from build123d import *

# Parameters (mm, degrees)
IZIM2_R                           = 5
KES_EKSTR_ZYON3_DEPTH             = 12
KES_EKSTR_ZYON3_TAPER             = -20
KES_EKSTR_ZYON3_OTHER_WAY_DEPTH   = 12
KES_EKSTR_ZYON3_OTHER_WAY_DRAFT   = -20
DAIRESEL_KAPLAMA1_COUNT           = 5
DAIRESEL_KAPLAMA1_COPY_1_SKETCH_R = 5
DAIRESEL_KAPLAMA1_COPY_1_DEPTH    = 12
DAIRESEL_KAPLAMA1_COPY_1_DRAFT    = -20
DAIRESEL_KAPLAMA1_COPY_2_SKETCH_R = 5
DAIRESEL_KAPLAMA1_COPY_2_DEPTH    = 12
DAIRESEL_KAPLAMA1_COPY_2_DRAFT    = -20
DAIRESEL_KAPLAMA1_COPY_3_SKETCH_R = 5
DAIRESEL_KAPLAMA1_COPY_3_DEPTH    = 12
DAIRESEL_KAPLAMA1_COPY_3_DRAFT    = -20
DAIRESEL_KAPLAMA1_COPY_4_SKETCH_R = 5
DAIRESEL_KAPLAMA1_COPY_4_DEPTH    = 12
DAIRESEL_KAPLAMA1_COPY_4_DRAFT    = -20
DAIRESEL_KAPLAMA1_COPY_5_SKETCH_R = 5
DAIRESEL_KAPLAMA1_COPY_5_DEPTH    = 12
DAIRESEL_KAPLAMA1_COPY_5_DRAFT    = -20
DAIRESEL_KAPLAMA1_COPY_6_SKETCH_R = 5
DAIRESEL_KAPLAMA1_COPY_6_DEPTH    = 12
DAIRESEL_KAPLAMA1_COPY_6_DRAFT    = -20
DAIRESEL_KAPLAMA1_COPY_7_SKETCH_R = 5
DAIRESEL_KAPLAMA1_COPY_7_DEPTH    = 12
DAIRESEL_KAPLAMA1_COPY_7_DRAFT    = -20
DAIRESEL_KAPLAMA1_COPY_8_SKETCH_R = 5
DAIRESEL_KAPLAMA1_COPY_8_DEPTH    = 12
DAIRESEL_KAPLAMA1_COPY_8_DRAFT    = -20


with BuildPart() as part:
    # Çizim1 → Döndür1 (revolve)
    with BuildSketch(Plane.XY, mode=Mode.PRIVATE) as d_nd_r1_sk:
        Polygon((-10.136635142, 50), (-0.136635142, 40), (9.863364858, 50), (11.863364858, 50), (11.863364858, 20), (14.863364858, 20), (14.863364858, 15), (11.863364858, 15), (-12.136635142, 15), (-15.136635142, 15), (-15.136635142, 20), (-12.136635142, 20), (-12.136635142, 50), align=None)
    revolve(d_nd_r1_sk.sketch.rotate(Axis((-17.676704828, 0, 0), (1, 0, 0)), 90), axis=Axis((-17.676704828, 0, 0), (1, 0, 0)))

    # Çizim2 → Kes-Ekstrüzyon3 (cut)
    with BuildSketch(Plane(origin=(-0.136635142, 0, 0), x_dir=(0, 0, -1), z_dir=(1, 0, 0))):
        with Locations((0, 30)):
            Circle(IZIM2_R)
    kes_ekstr_zyon3 = extrude(amount=-KES_EKSTR_ZYON3_DEPTH, taper=KES_EKSTR_ZYON3_TAPER, mode=Mode.SUBTRACT)


with BuildPart() as kes_ekstr_zyon3_other_way_tool:
    # Çizim2 → Kes-Ekstrüzyon3 other way (with draft: the straight prism first)
    with BuildSketch(Plane(origin=(-0.136635142, 0, 0), x_dir=(0, 0, -1), z_dir=(1, 0, 0))):
        with Locations((0, 30)):
            Circle(IZIM2_R)
    extrude(amount=KES_EKSTR_ZYON3_OTHER_WAY_DEPTH)
    # Kes-Ekstrüzyon3 other way: the draft: its side faces are tilted about the plane it starts from
    kes_ekstr_zyon3_other_way_sides = [kes_ekstr_zyon3_other_way_tool.faces().sort_by_distance(p)[0] for p in [
        (5.863364858, 30, 5),
    ]]
    draft(kes_ekstr_zyon3_other_way_sides, Plane(origin=(-0.136635142, 0, 0), x_dir=(0, 0, -1), z_dir=(1, 0, 0)), KES_EKSTR_ZYON3_OTHER_WAY_DRAFT)


with BuildPart() as part_1:
    add(part.part)

    # Kes-Ekstrüzyon3 other way: cut by kes_ekstr_zyon3_other_way_tool
    add(kes_ekstr_zyon3_other_way_tool.part, mode=Mode.SUBTRACT)

    # Dairesel Kaplama1: Kes-Ekstrüzyon3 ×5 about axis
    dairesel_kaplama1_axis = Axis((0, 0, 0), (1, 0, 0))
    for i in range(1, DAIRESEL_KAPLAMA1_COUNT):
        add(kes_ekstr_zyon3.rotate(dairesel_kaplama1_axis, i * 360 / DAIRESEL_KAPLAMA1_COUNT), mode=Mode.SUBTRACT)


with BuildPart() as dairesel_kaplama1_copy_1_tool:
    # Dairesel Kaplama1 copy 1 sketch → Dairesel Kaplama1 copy 1 (with draft: the straight prism first)
    with BuildSketch(Plane(origin=(-0.136635142, 0, 0), x_dir=(0, 0.9510565162951535, -0.30901699437494745), z_dir=(1, 0, 0))):
        with Locations((0, 30)):
            Circle(DAIRESEL_KAPLAMA1_COPY_1_SKETCH_R)
    extrude(amount=DAIRESEL_KAPLAMA1_COPY_1_DEPTH)
    # Dairesel Kaplama1 copy 1: the draft: its side faces are tilted about the plane it starts from
    dairesel_kaplama1_copy_1_sides = [dairesel_kaplama1_copy_1_tool.faces().sort_by_distance(p)[0] for p in [
        (5.863364858, 4.51522725, 30.076780461),
    ]]
    draft(dairesel_kaplama1_copy_1_sides, Plane(origin=(-0.136635142, 0, 0), x_dir=(0, 0.9510565162951535, -0.30901699437494745), z_dir=(1, 0, 0)), DAIRESEL_KAPLAMA1_COPY_1_DRAFT)


with BuildPart() as part_2:
    add(part_1.part)

    # Dairesel Kaplama1 copy 1: cut by dairesel_kaplama1_copy_1_tool
    add(dairesel_kaplama1_copy_1_tool.part, mode=Mode.SUBTRACT)


with BuildPart() as dairesel_kaplama1_copy_2_tool:
    # Dairesel Kaplama1 copy 2 sketch → Dairesel Kaplama1 copy 2 (with draft: the straight prism first)
    with BuildSketch(Plane(origin=(-0.136635142, 0, 0), x_dir=(0, 0.5877852522924732, 0.8090169943749473), z_dir=(1, 0, 0))):
        with Locations((0, 30)):
            Circle(DAIRESEL_KAPLAMA1_COPY_2_SKETCH_R)
    extrude(amount=DAIRESEL_KAPLAMA1_COPY_2_DEPTH)
    # Dairesel Kaplama1 copy 2: the draft: its side faces are tilted about the plane it starts from
    dairesel_kaplama1_copy_2_sides = [dairesel_kaplama1_copy_2_tool.faces().sort_by_distance(p)[0] for p in [
        (5.863364858, -27.209436093, 13.588472597),
    ]]
    draft(dairesel_kaplama1_copy_2_sides, Plane(origin=(-0.136635142, 0, 0), x_dir=(0, 0.5877852522924732, 0.8090169943749473), z_dir=(1, 0, 0)), DAIRESEL_KAPLAMA1_COPY_2_DRAFT)


with BuildPart() as part_3:
    add(part_2.part)

    # Dairesel Kaplama1 copy 2: cut by dairesel_kaplama1_copy_2_tool
    add(dairesel_kaplama1_copy_2_tool.part, mode=Mode.SUBTRACT)


with BuildPart() as dairesel_kaplama1_copy_3_tool:
    # Dairesel Kaplama1 copy 3 sketch → Dairesel Kaplama1 copy 3 (with draft: the straight prism first)
    with BuildSketch(Plane(origin=(-0.136635142, 0, 0), x_dir=(0, -0.587785252292473, 0.8090169943749476), z_dir=(1, 0, 0))):
        with Locations((0, 30)):
            Circle(DAIRESEL_KAPLAMA1_COPY_3_SKETCH_R)
    extrude(amount=DAIRESEL_KAPLAMA1_COPY_3_DEPTH)
    # Dairesel Kaplama1 copy 3: the draft: its side faces are tilted about the plane it starts from
    dairesel_kaplama1_copy_3_sides = [dairesel_kaplama1_copy_3_tool.faces().sort_by_distance(p)[0] for p in [
        (5.863364858, -21.33158357, -21.678642541),
    ]]
    draft(dairesel_kaplama1_copy_3_sides, Plane(origin=(-0.136635142, 0, 0), x_dir=(0, -0.587785252292473, 0.8090169943749476), z_dir=(1, 0, 0)), DAIRESEL_KAPLAMA1_COPY_3_DRAFT)


with BuildPart() as part_4:
    add(part_3.part)

    # Dairesel Kaplama1 copy 3: cut by dairesel_kaplama1_copy_3_tool
    add(dairesel_kaplama1_copy_3_tool.part, mode=Mode.SUBTRACT)


with BuildPart() as dairesel_kaplama1_copy_4_tool:
    # Dairesel Kaplama1 copy 4 sketch → Dairesel Kaplama1 copy 4 (with draft: the straight prism first)
    with BuildSketch(Plane(origin=(-0.136635142, 0, 0), x_dir=(0, -0.9510565162951536, -0.30901699437494723), z_dir=(1, 0, 0))):
        with Locations((0, 30)):
            Circle(DAIRESEL_KAPLAMA1_COPY_4_SKETCH_R)
    extrude(amount=DAIRESEL_KAPLAMA1_COPY_4_DEPTH)
    # Dairesel Kaplama1 copy 4: the draft: its side faces are tilted about the plane it starts from
    dairesel_kaplama1_copy_4_sides = [dairesel_kaplama1_copy_4_tool.faces().sort_by_distance(p)[0] for p in [
        (5.863364858, 14.025792413, -26.986610517),
    ]]
    draft(dairesel_kaplama1_copy_4_sides, Plane(origin=(-0.136635142, 0, 0), x_dir=(0, -0.9510565162951536, -0.30901699437494723), z_dir=(1, 0, 0)), DAIRESEL_KAPLAMA1_COPY_4_DRAFT)


with BuildPart() as part_5:
    add(part_4.part)

    # Dairesel Kaplama1 copy 4: cut by dairesel_kaplama1_copy_4_tool
    add(dairesel_kaplama1_copy_4_tool.part, mode=Mode.SUBTRACT)


with BuildPart() as dairesel_kaplama1_copy_5_tool:
    # Dairesel Kaplama1 copy 5 sketch → Dairesel Kaplama1 copy 5 (with draft: the straight prism first)
    with BuildSketch(Plane(origin=(-0.136635142, 0, 0), x_dir=(0, 0.9510565162951535, -0.30901699437494745), z_dir=(1, 0, 0))):
        with Locations((0, 30)):
            Circle(DAIRESEL_KAPLAMA1_COPY_5_SKETCH_R)
    extrude(amount=DAIRESEL_KAPLAMA1_COPY_5_DEPTH)
    # Dairesel Kaplama1 copy 5: the draft: its side faces are tilted about the plane it starts from
    dairesel_kaplama1_copy_5_sides = [dairesel_kaplama1_copy_5_tool.faces().sort_by_distance(p)[0] for p in [
        (5.863364858, 4.51522725, 30.076780461),
    ]]
    draft(dairesel_kaplama1_copy_5_sides, Plane(origin=(-0.136635142, 0, 0), x_dir=(0, 0.9510565162951535, -0.30901699437494745), z_dir=(1, 0, 0)), DAIRESEL_KAPLAMA1_COPY_5_DRAFT)


with BuildPart() as part_6:
    add(part_5.part)

    # Dairesel Kaplama1 copy 5: cut by dairesel_kaplama1_copy_5_tool
    add(dairesel_kaplama1_copy_5_tool.part, mode=Mode.SUBTRACT)


with BuildPart() as dairesel_kaplama1_copy_6_tool:
    # Dairesel Kaplama1 copy 6 sketch → Dairesel Kaplama1 copy 6 (with draft: the straight prism first)
    with BuildSketch(Plane(origin=(-0.136635142, 0, 0), x_dir=(0, 0.5877852522924732, 0.8090169943749473), z_dir=(1, 0, 0))):
        with Locations((0, 30)):
            Circle(DAIRESEL_KAPLAMA1_COPY_6_SKETCH_R)
    extrude(amount=DAIRESEL_KAPLAMA1_COPY_6_DEPTH)
    # Dairesel Kaplama1 copy 6: the draft: its side faces are tilted about the plane it starts from
    dairesel_kaplama1_copy_6_sides = [dairesel_kaplama1_copy_6_tool.faces().sort_by_distance(p)[0] for p in [
        (5.863364858, -27.209436093, 13.588472597),
    ]]
    draft(dairesel_kaplama1_copy_6_sides, Plane(origin=(-0.136635142, 0, 0), x_dir=(0, 0.5877852522924732, 0.8090169943749473), z_dir=(1, 0, 0)), DAIRESEL_KAPLAMA1_COPY_6_DRAFT)


with BuildPart() as part_7:
    add(part_6.part)

    # Dairesel Kaplama1 copy 6: cut by dairesel_kaplama1_copy_6_tool
    add(dairesel_kaplama1_copy_6_tool.part, mode=Mode.SUBTRACT)


with BuildPart() as dairesel_kaplama1_copy_7_tool:
    # Dairesel Kaplama1 copy 7 sketch → Dairesel Kaplama1 copy 7 (with draft: the straight prism first)
    with BuildSketch(Plane(origin=(-0.136635142, 0, 0), x_dir=(0, -0.587785252292473, 0.8090169943749476), z_dir=(1, 0, 0))):
        with Locations((0, 30)):
            Circle(DAIRESEL_KAPLAMA1_COPY_7_SKETCH_R)
    extrude(amount=DAIRESEL_KAPLAMA1_COPY_7_DEPTH)
    # Dairesel Kaplama1 copy 7: the draft: its side faces are tilted about the plane it starts from
    dairesel_kaplama1_copy_7_sides = [dairesel_kaplama1_copy_7_tool.faces().sort_by_distance(p)[0] for p in [
        (5.863364858, -21.33158357, -21.678642541),
    ]]
    draft(dairesel_kaplama1_copy_7_sides, Plane(origin=(-0.136635142, 0, 0), x_dir=(0, -0.587785252292473, 0.8090169943749476), z_dir=(1, 0, 0)), DAIRESEL_KAPLAMA1_COPY_7_DRAFT)


with BuildPart() as part_8:
    add(part_7.part)

    # Dairesel Kaplama1 copy 7: cut by dairesel_kaplama1_copy_7_tool
    add(dairesel_kaplama1_copy_7_tool.part, mode=Mode.SUBTRACT)


with BuildPart() as dairesel_kaplama1_copy_8_tool:
    # Dairesel Kaplama1 copy 8 sketch → Dairesel Kaplama1 copy 8 (with draft: the straight prism first)
    with BuildSketch(Plane(origin=(-0.136635142, 0, 0), x_dir=(0, -0.9510565162951536, -0.30901699437494723), z_dir=(1, 0, 0))):
        with Locations((0, 30)):
            Circle(DAIRESEL_KAPLAMA1_COPY_8_SKETCH_R)
    extrude(amount=DAIRESEL_KAPLAMA1_COPY_8_DEPTH)
    # Dairesel Kaplama1 copy 8: the draft: its side faces are tilted about the plane it starts from
    dairesel_kaplama1_copy_8_sides = [dairesel_kaplama1_copy_8_tool.faces().sort_by_distance(p)[0] for p in [
        (5.863364858, 14.025792413, -26.986610517),
    ]]
    draft(dairesel_kaplama1_copy_8_sides, Plane(origin=(-0.136635142, 0, 0), x_dir=(0, -0.9510565162951536, -0.30901699437494723), z_dir=(1, 0, 0)), DAIRESEL_KAPLAMA1_COPY_8_DRAFT)


with BuildPart() as part_9:
    add(part_8.part)

    # Dairesel Kaplama1 copy 8: cut by dairesel_kaplama1_copy_8_tool
    add(dairesel_kaplama1_copy_8_tool.part, mode=Mode.SUBTRACT)


solid = part_9.part
The listing builds one solid part. Answer for the finished solid, in the listing's coordinates (mm). A direction names the side the tool comes from. Coordinates: 2 decimals unless noted, no trailing zeros. Order: outer loops, then holes, each group sorted by start corner. A loop starts at its lowest first (then second) coordinate and runs counter-clockwise, first axis right, second up.
Q1. Which of the six approach directions +Z, -Z, +X, -X, +Y, -Y give full straight-line access (tool end or side, diameter ignored) to faces 4 (the face through (3.11, 4.86, -24.2)), 5 (the face through (-12.137, -1, -22)), 6 (the face through (-0.622, -12.161, 38.616))?
Q2. Given P1, Ø1, axis at x = -5, z = 8, coming from the +Y side; P2, Ø8, axis at x = 8.5, y = 29.5, coming from the -Z side; P3, Ø12, axis at x = -1, y = 20.5, coming from the +Z side, each flat-ended and moving along its own axis, determine where each tip first touches the part or whether it passes through.
Q3. A cutting plane is placed at A-A, the plane z = 0. Write down the section's boundary in (x, y), and give its area (3 significant figures).
Q4. A cutting plane is placed at B-B, the plane x = 7.75. Write down the section's boundary in (y, z).
Q5. Consider line 1 (Y direction, x = 3.75, z = 0); line 2 (Z direction, x = -8.5, y = 13); line 3 (Y direction, x = 5.75, z = 12). Determine where each line is inside the solid, lowest interval first.
Q6. For a pull along Y with two mould halves and no side action, classify faces 1 (the face through (3.113, 23.964, 1.34)), 2 (the face through (13.38, -0.88, -19.98)), 3 (the face through (11.863, -1, 22)) as pulls with the +Y half, pulls with the -Y half, needs draft (parallel to the pull), parting line crosses it, or undercut.
Answers follow:
1. face 4: +X
1. face 5: -X
1. face 6: none
2. P1: stops at y = 44.66
2. P2: stops at z = -42.87
2. P3: stops at z = 42.69
3. outline: (-15.14, -20) - (-12.14, -20) - (-12.14, -50) - (-10.14, -50) - (-0.14, -40) - (9.86, -50) - (11.86, -50) - (11.86, -20) - (14.86, -20) - (14.86, -15) - (-15.14, -15) - close; (-15.14, 15) - (14.86, 15) - (14.86, 20) - (11.86, 20) - (11.86, 20.63) - (-0.14, 25) - (-12.14, 20.63) - (-12.14, 20) - (-15.14, 20) - close; (-12.14, 39.37) - (-0.14, 35) - (11.86, 39.37) - (11.86, 50) - (9.86, 50) - (-0.14, 40) - (-10.14, 50) - (-12.14, 50) - close
3. area: 1,200 mm2
4. outline: circle Ø95.77 at (0, 0); hole circle Ø15.74 at (-24.27, -17.63); hole circle Ø15.74 at (-24.27, 17.63); hole circle Ø30 at (0, 0); hole circle Ø15.74 at (9.27, -28.53); hole circle Ø15.74 at (9.27, 28.53); hole circle Ø15.74 at (30, 0)
5. line 1: y = -43.89 to -15, 15 to 23.59, 36.41 to 43.89
5. line 2: z = -46.58 to -35.66, -21.4 to -7.48, 7.48 to 21.4, 35.66 to 46.58
5. line 3: y = -44.29 to -28.66, -19.88 to -9, 9 to 44.29
6. face 1: undercut
6. face 2: parting line crosses it
6. face 3: needs draft
